from build123d import *

# Parameters (mm, degrees)
F0_R     = 11.05
F1_DEPTH = 22
F2_D     = 1.66116


with BuildPart() as f1:
    # F0 (on Top) → F1 (new body)
    with BuildSketch(Plane.XY):
        Circle(F0_R)
    extrude(amount=-F1_DEPTH)

    # F2 (through all)
    with Locations(Plane.XY):
        with Locations((0, 5), (-5, 5), (-5, 0), (-5, -5), (0, -5), (5, -5), (5, 0), (5, 5), (0, 0)):
            Hole(F2_D / 2)


solid = f1.part
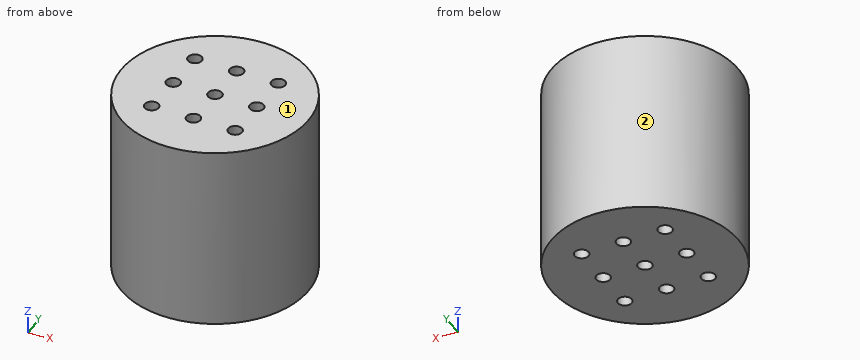
Geometry check sheet. Reference: the model listing, model coordinates, mm. Face numbers are marked on the shaded views. Give positions to 0.01 mm unless a question says otherwise; leave off trailing zeros. Order: outer loops, then holes, each group sorted by start corner. A loop starts at its lowest first (then second) coordinate and runs counter-clockwise, first axis right, second up.
1. Draft check along Y on the marked faces 1 and 2. Enter one of: pulls with the +Y half, pulls with the -Y half, needs draft (parallel to the pull), parting line crosses it, or undercut.
Completed:
face 1: needs draft
face 2: parting line crosses it
2. Sectioned sample at D-D (x = 9.75). Record the boundary of the cut face in (y, z).
Completed:
outline: (-5.2, -22) - (5.2, -22) - (5.2, 0) - (-5.2, 0) - close
3. Scan lines: line 1 (Y direction, x = 0, z = -13.5); line 2 (Y direction, x = 4.25, z = -10); line 3 (X direction, y = -5.25, z = -9). Record each from-to range of solid material in increasing order.
Completed:
line 1: y = -11.05 to -5.83, -4.17 to -0.83, 0.83 to 4.17, 5.83 to 11.05
line 2: y = -10.2 to -5.36, -4.64 to -0.36, 0.36 to 4.64, 5.36 to 10.2
line 3: x = -9.72 to -5.79, -4.21 to -0.79, 0.79 to 4.21, 5.79 to 9.72
4. Depth check by flat-ended pin: pin 1 (1 mm diameter, centred on y = 5, z = -11, fed in from +X); pin 2 (1 mm diameter, centred on x = 8, z = -11, fed in from -Y); pin 3 (6 mm diameter, centred on x = -5.5, z = -15.5, fed in from -Y). Enter the tip coordinate at first touch or a pass-through.
Completed:
pin 1: stops at x = 10.09
pin 2: stops at y = -8.11
pin 3: stops at y = -10.76
5. Sectioned sample at B-B (z = -18.75). State how many separate pieces and enclosed holes the cut face has, then the cut area to 3 significant figures.
Completed:
separate pieces: 1
enclosed holes: 9
area: 364 mm2
6. Sectioned sample at A-A (y = 0). Record the boundary of the cut face in (x, z).
Completed:
outline: (-11.05, -22) - (-5.83, -22) - (-5.83, 0) - (-11.05, 0) - close; (-4.17, -22) - (-0.83, -22) - (-0.83, 0) - (-4.17, 0) - close; (0.83, -22) - (4.17, -22) - (4.17, 0) - (0.83, 0) - close; (5.83, -22) - (11.05, -22) - (11.05, 0) - (5.83, 0) - close
